from build123d import *

# Parameters (mm, degrees)
F0_W      = 1524
F0_H      = 304.8
F1_DEPTH  = 25.4
F1_TAPER  = -3
F1_FACE_W = 1526.6623151876
F1_FACE_H = 307.4623151876
F3_DEPTH  = 25.4
F3_TAPER  = -3
F4_W      = 36.3832712173
F4_H      = 308.6890354753
F5_DEPTH  = 609.6


# Not quite as in the source:
# - a feature names something its author has since deleted; it is built from what else it names


with BuildPart() as f1:
    # F0 (on Top) → F1 (new body)
    with BuildSketch(Plane.XY):
        with Locations((-1.6607679427, -79.0239475151)):
            Rectangle(F0_W, F0_H)
    extrude(amount=F1_DEPTH, taper=F1_TAPER)

    # F1_face (on face) → F3 (join)
    with BuildSketch(Plane(origin=(-1.6607679427, -79.0239475151, 25.4), x_dir=(1, 0, 0), z_dir=(0, 0, 1))):
        Rectangle(F1_FACE_W, F1_FACE_H)
    extrude(amount=F3_DEPTH, taper=F3_TAPER)

    # F4 (on Top) → F5 (join)
    with BuildSketch(Plane.XY):
        with Locations((-783.7679982185, -78.7090621889)):
            Rectangle(F4_W, F4_H)
    extrude(amount=F5_DEPTH)


solid = f1.part
Verification items for the finished model (mm, model axes). A direction names the side the tool comes from. Coordinates: 2 decimals unless noted, no trailing zeros. Order: outer loops, then holes, each group sorted by start corner. A loop starts at its lowest first (then second) coordinate and runs counter-clockwise, first axis right, second up. Notation, with made-up numbers: M -10,84 L 22,84 A16 cw 22,104 Z; hole C -15,59 d11. An arc over 180 degrees is marked long. Return JSON: item names as keys, results as strings.
1) Access from +Z, -Z, +X, -X, +Y, -Y to the whole of each face (thin tool, end or side, straight path). Record for faces 5 (the flat face through (-765.576, -81, 326)), 6 (the flat face through (-784, -77, 0)), 7 (the flat face through (9.045, 74.726, 25.756)).
Answer list:
{"face 5": "+Z, +X, +Y, -Y", "face 6": "-Z, +X, -X, +Y, -Y", "face 7": "-Z, +X, +Y"}
2) Release check for a two-part mould opening along Z. For faces 1 (the flat face through (-784, -77, 609.6)), 2 (the flat face through (-765.576, -81, 21)), 3 (the flat face through (-784, -233.054, 301)), 4 (the flat face through (-12.366, -232.774, 25.756)) record: +Z half, -Z half, draft (parallel to the pull), parting line (faces both ways), or undercut.
Answer list:
{"face 1": "+Z half", "face 2": "undercut", "face 3": "draft", "face 4": "-Z half"}
3) Thickness scan on L1, parallel to X at y = -36, z = 67.5; L2, parallel to Z at x = 262, y = -108.5; L3, parallel to Y at x = 618, z = 33.5. Record the ranges inside material, lowest first. Write a range as [from, to].
Answer list:
{"L1": "[-801.96, -765.58]", "L2": "[0, 50.8]", "L3": "[-233.18, 75.13]"}
4) Gauge pin test, flat ends, axial feed: pin 1 (11 mm diameter, centred on x = -785, z = 322.5, fed in from +Y); pin 2 (12 mm diameter, centred on x = -137.5, y = -11, fed in from -Z); pin 3 (2 mm diameter, centred on y = -39.5, z = 416.5, fed in from +X); pin 4 (10 mm diameter, centred on x = 192.5, y = -56.5, fed in from +Z). Record the tip position at first contact, or that the pin passes through.
Answer list:
{"pin 1": "y = 75.64", "pin 2": "z = 0", "pin 3": "x = -765.58", "pin 4": "z = 50.8"}
5) Cross-section at B-B, the plane x = -676.5. Record the boundary of the cut face in (y, z).
Answer list:
{"outline": "M -234.09,50.8 L -231.42,0 L 73.38,0 L 76.04,50.8 Z"}
6) Cross-section at C-C, the plane y = -107.5. Record the boundary of the cut face in (x, z), and give its area (3 significant figures).
Answer list:
{"outline": "M -801.96,0 L -765.58,0 L -765.58,36.55 L -763.66,0 L 760.34,0 L 763,50.8 L -765.58,50.8 L -765.58,609.6 L -801.96,609.6 Z", "area": "99,700 mm2"}
7) Cross-section at A-A, the plane z = 462.5. Record the boundary of the cut face in (x, y).
Answer list:
{"outline": "M -801.96,-233.05 L -765.58,-233.05 L -765.58,75.64 L -801.96,75.64 Z"}
